Could you check a few things on this model? Use its own coordinates, in mm. Round coordinates to 2 decimals unless told otherwise and drop trailing zeros. Order: outer loops, then holes, each group sorted by start corner. A loop starts at its lowest first (then second) coordinate and runs counter-clockwise, first axis right, second up. Notation, with made-up numbers: M -28,50.25 L 4,50.25 A31 cw 4,88.25 Z; hole C 36,51 d8. An arc over 180 degrees is marked long. Write each question's results on one line, items separated by ' | '. Start each with the question number.
1. Suppose I cut it at C-C on x = -42. Write out the boundary of the cut face in (y, z), and give its area (3 significant figures).
2. Please list where these lines run through material, in increasing order: L1, parallel to Z at x = 0.5, y = 2.9; L2, parallel to Z at x = -42.5, y = 2.9.
3. Suppose I cut it at A-A on y = 1.55. Write out the boundary of the cut face in (x, z) (3 decimals), and give its area (3 significant figures).
4. Suppose I cut it at B-B on x = 17. Write out the boundary of the cut face in (y, z).
from build123d import *

# Parameters (mm, degrees)
SKETCH1_W           = 57.15
SKETCH1_H           = 12.7
BOSS_EXTRUDE1_DEPTH = 3.2


with BuildPart() as part:
    # Sketch1 → Boss-Extrude1 (new body)
    with BuildSketch(Plane(origin=(0, 0, 0), x_dir=(1, 0, 0), z_dir=(0, 1, 0))):
        with BuildLine():
            Line((-28.575, -6.35), (-28.575, 6.35))
            ThreePointArc((-28.575, 6.35), (-36.352129933, 7.152195105), (-43.801765087, 9.525))
            Line((-43.801765087, 9.525), (-82.55, 9.525))
            Line((-82.55, 9.525), (-82.55, -9.525))
            Line((-82.55, -9.525), (-43.801765087, -9.525))
            ThreePointArc((-43.801765087, -9.525), (-36.352129933, -7.152195105), (-28.575, -6.35))
        make_face()
        Rectangle(SKETCH1_W, SKETCH1_H)
        with BuildLine():
            ThreePointArc((43.801765087, 9.525), (36.352129933, 7.152195105), (28.575, 6.35))
            Line((28.575, 6.35), (28.575, -6.35))
            ThreePointArc((28.575, -6.35), (36.352129933, -7.152195105), (43.801765087, -9.525))
            Line((43.801765087, -9.525), (82.55, -9.525))
            Line((82.55, -9.525), (82.55, 9.525))
            Line((82.55, 9.525), (43.801765087, 9.525))
        make_face()
    extrude(amount=BOSS_EXTRUDE1_DEPTH)


solid = part.part
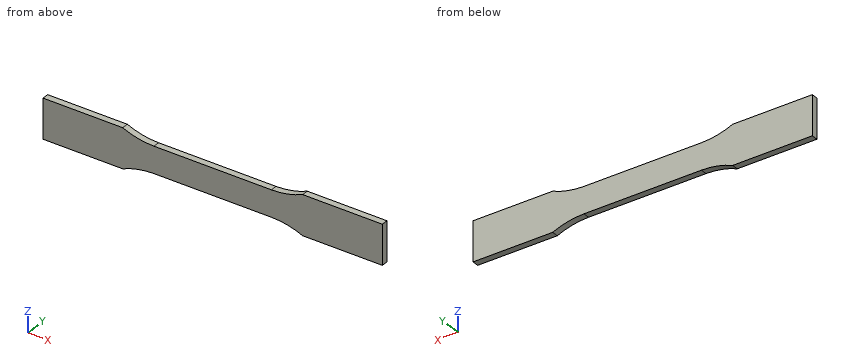
Filled sheet:
1) outline: M 0,-8.79 L 3.2,-8.79 L 3.2,8.79 L 0,8.79 Z | area: 56.3 mm^2
2) L1: z = -6.35 to 6.35 | L2: z = -8.99 to 8.99
3) outline: M -82.55,-9.525 L -43.802,-9.525 A38.1 cw -28.575,-6.35 L 28.575,-6.35 A38.1 cw 43.802,-9.525 L 82.55,-9.525 L 82.55,9.525 L 43.802,9.525 A38.1 cw 28.575,6.35 L -28.575,6.35 A38.1 cw -43.802,9.525 L -82.55,9.525 Z | area: 2,650 mm^2
4) outline: M 0,-6.35 L 3.2,-6.35 L 3.2,6.35 L 0,6.35 Z
